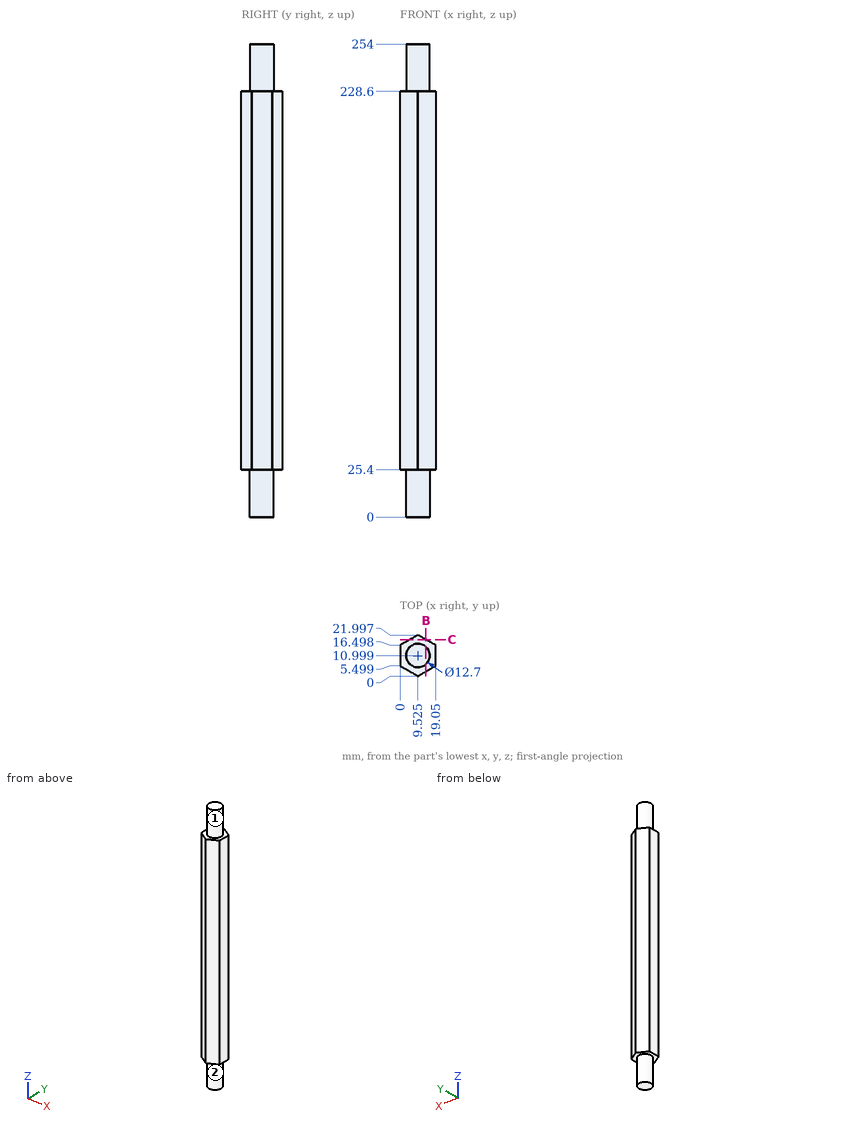
Design review of the part shown in the three views and the two pictorial views. Dimensions are in mm from the part's minimum x, y and z. A direction names the side the tool comes from. Coordinates: 2 decimals unless noted, no trailing zeros. Order: outer loops, then holes, each group sorted by start corner. A loop starts at its lowest first (then second) coordinate and runs counter-clockwise, first axis right, second up.
Item 1: Take a section at C-C, the plane y = 19.5. Write out the cut boundary in (x, z), then the cut area to 3 significant figures.
Item 2: For pin 1 Ø4 at (x, z) = (17, 40.5) entering from +Y (1 decimal); pin 2 Ø1.5 at (y, z) = (18, 175.5) entering from -X (1 decimal); pin 3 Ø6 at (x, z) = (11.5, 91.5) entering from -Y, all flat-tipped, find the tip position at first contact; note any pin that passes through.
Item 3: For line 1 (Y direction, x = 1.5, z = 211.5) (1 decimal); line 2 (Z direction, x = 14, y = 5); line 3 (X direction, y = 17.5, z = 60.5) (1 decimal), list the stretches that pass through material, from the lowest coordinate up.
Item 4: Take a section at B-B, the plane x = 13.75. Write out the cut boundary in (y, z).
Item 5: For the marked faces 1 and 2, list the 3-axis set-ups (+Z, -Z, +X, -X, +Y, -Y) from which the entire face can be reached by the end or side of a thin tool; tool diameter is ignored.
The answers:
1. outline: (5.2, 25.4) - (13.85, 25.4) - (13.85, 228.6) - (5.2, 228.6) - close
1. area: 1,760 mm2
2. pin 1: stops at y = 18.8
2. pin 2: stops at x = 1.3
2. pin 3: stops at y = 0
3. line 1: y = 4.6 to 17.4
3. line 2: z = 25.4 to 228.6
3. line 3: x = 1.7 to 17.3
4. outline: (2.44, 25.4) - (6.26, 25.4) - (6.26, 0) - (15.74, 0) - (15.74, 25.4) - (19.56, 25.4) - (19.56, 228.6) - (15.74, 228.6) - (15.74, 254) - (6.26, 254) - (6.26, 228.6) - (2.44, 228.6) - close
5. face 1: +Z
5. face 2: -Z
